```python
from build123d import *

# Parameters (mm, degrees)
F3_D     = 50
F3_DEPTH = 50
F3_TIP   = 15.0215154757


with BuildPart() as f1:
    # F0 (on Front) → F1 (revolve)
    with BuildSketch(Plane.XZ):
        Polygon((-64.8, 0), (0, 0), (0, 150), (-64.8, 150), (-64.8, 130), (-44.8, 130), (-44.8, 110), (-64.8, 110), align=None)
    revolve(axis=Axis((0, 0, 75), (0, 0, -1)))

    # F3
    with Locations(Plane(origin=(0, 0, 0), x_dir=(1, 0, 0), z_dir=(0, 0, -1))):
        with Locations((0, 0)):
            Hole(F3_D / 2, depth=F3_DEPTH)
            with Locations((0, 0, -(F3_DEPTH + F3_TIP / 2))):  # 118° drill point
                Cone(0, F3_D / 2, F3_TIP, mode=Mode.SUBTRACT)


solid = f1.part
```
The listing builds one solid part. Answer for the finished solid, in the listing's coordinates (mm). A direction names the side the tool comes from. Coordinates: 2 decimals unless noted, no trailing zeros. Order: outer loops, then holes, each group sorted by start corner. A loop starts at its lowest first (then second) coordinate and runs counter-clockwise, first axis right, second up. Notation, with made-up numbers: M 10,-28 L 43,-28 A11 cw 43,-19 Z; hole C 72,43 d11. An arc over 180 degrees is marked long. Answer as a JSON object with one key per item and string values. Group by question number.
1. A tool of negligible diameter and unlimited length cuts with its end or side. For faces 4 (the flat face through (-42.3, 15.3, 130)), 5 (the flat face through (1, -28, 0)), 6 (the cylindrical face through (-23.846, -7.509, 25.35)), from which of +Z, -Z, +X, -X, +Y, -Y can it reach the whole face along a straight path? Write none if from no direction.
2. Section B-B on z = 11 is taken. Write down the section's boundary in (x, y), then the cut area to 3 significant figures.
3. Straight lines are drawn through the part: line 1 (Y direction, x = 0, z = 26); line 2 (Z direction, x = -21.5, y = 48); line 3 (X direction, y = -6, z = 55.5). For each, find the intervals that lie inside material, in ascending order.
4. Section A-A on y = 54.5 is taken. Write down the section's boundary in (x, z).
5. Flat-ended cylindrical pins translate along their axes: P1, Ø1, axis at y = 52, z = 73.5, coming from the -X side; P2, Ø3, axis at x = -27.5, z = 49.5, coming from the +Y side; P3, Ø5, axis at y = -32, z = 130, coming from the -X side. Find the tip coordinate at first contact, or state that the pin passes through.
6. Determine the mould class of faces 1 (the cylindrical face through (14.05, -63.26, 54.23)), 2 (the flat face through (-1, 1, 150)), 3 (the cylindrical face through (44.757, 1.97, 119.86)) for opening direction Z: released by +Z, released by -Z, zero draft, split by the parting line, or undercut.
7. Section C-C on z = 141 is taken. Write down the section's boundary in (x, y).
Values follow:
{
 "1": {"face 4": "none", "face 5": "-Z, +X, -X, +Y, -Y", "face 6": "-Z"},
 "2": {"outline": "C 0,0 d129.6; hole C 0,0 d50", "area": "11,200 mm2"},
 "3": {"line 1": "-64.8 to -25, 25 to 64.8", "line 2": "0 to 110, 130 to 150", "line 3": "-64.52 to -14.67, 14.67 to 64.52"},
 "4": {"outline": "M -35.05,0 L 35.05,0 L 35.05,110 L -35.05,110 Z; M -35.05,130 L 35.05,130 L 35.05,150 L -35.05,150 Z"},
 "5": {"P1": "x = -39.33", "P2": "y = 59.36", "P3": "x = -57.7"},
 "6": {"face 1": "zero draft", "face 2": "released by +Z", "face 3": "undercut"},
 "7": {"outline": "C 0,0 d129.6"}
}
